Check sheet for the modelled part. Datum: model origin and axes. Units: mm. Face numbers are marked on the shaded views. Coordinates: 2 decimals unless noted, no trailing zeros. Loops run counter-clockwise (first coordinate to the right, second up) from the corner with the lowest first, then second, coordinate; pieces in that order, holes last. Notation, with made-up numbers: M 53,23 L 110,23 A22 ccw 110,58 Z; hole C 45.25,-2 d3. An arc over 180 degrees is marked long. Use CSV: the item, a comma, the result in double quotes. Start each with the question number.
(1) Section check A-A on x = -12.5. Record the cut outline in (y, z).
(2) Section check B-B on x = 14.5. Record the cut outline in (y, z), and give its area (3 significant figures).
(3) Scan lines: line 1 (X direction, y = 22, z = -14.75); line 2 (X direction, y = 18.75, z = -12.75); line 3 (X direction, y = 19.5, z = -10.5). Record each from-to range of solid material in increasing order.
(4) Go/stop test with flat-tipped pins: pin 1 Ø2 at (x, z) = (-14.5, -13) entering from -Y; pin 2 Ø3 at (x, z) = (-8.5, -17) entering from +Y; pin 3 Ø1 at (x, z) = (-9.5, -15) entering from -Y. Record where each tip stops, or that it passes through.
(5) Draft check along Y on the marked faces 1, 2 and 3. Enter one of: pulls with the +Y half, pulls with the -Y half, needs draft (parallel to the pull), parting line crosses it, or undercut.
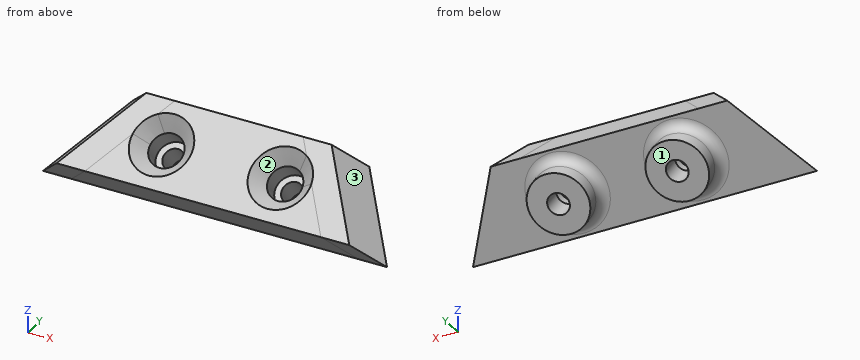
Autodesk Inventor part; units mm, degrees
ref_plane "作業平面2" through (-25, 27.5045, -21.6059) normal (0, -0.6427876, 0.7660444) x (1, 0, 0)
ref_plane "YZ Plane" through (0, 0, 0) normal (1, 0, 0) x (0, 1, 0)
ref_plane "XZ Plane" through (0, 0, 0) normal (0, 1, 0) x (-1, 0, 0)
sketch "スケッチ1" plane through (0, 0, 0) normal (0, 1, 0) x (-1, 0, 0)
  line L0 (28.2843, -28.2843) -> (0, 0)
  line L1 (0, 0) -> (-28.2843, -28.2843)
  line L2 (29.9813, -26.5872) -> (0, 3.3941)
  line L3 (0, 3.3941) -> (-29.9813, -26.5872)
  line L4 (28.2843, -28.2843) -> (29.9813, -26.5872)
  line L5 (-28.2843, -28.2843) -> (-29.9813, -26.5872)
  dimension "d0" = 40
  dimension "d1" = 2.4
extrude "押し出し1" add sketch "スケッチ1" along normal blind 50
sketch "スケッチ2" plane through (0, 0, 0) normal (1, 0, 0) x (0, 1, 0)
  line L0 (0, 3.3941) -> (31.9749, -34.7121)
  line L1 (0, 0) -> (0, -28.2843)
  line L2 (7.6604, 9.822) -> (39.6354, -28.2843)
  line L3 (0, 3.3941) -> (7.6604, 9.822)
  line L4 (39.6354, -28.2843) -> (31.9749, -34.7121)
  line L5 (0, -28.2843) -> (50, -28.2843)
  point P0 (26.5813, -28.2843)
  dimension "d4" = 40
  dimension "d5" = 10
extrude "押し出し2" cut sketch "スケッチ2" along normal mid plane 50 contours L3 L2 L5 L0 keep common part
ref_plane "作業平面1" through (0, 9.2239, 0.1802) normal (0, 0.7660444, 0.6427876) x (0.7938448, -0.3908923, 0.4658473)
sketch "スケッチ4" plane through (0, 9.2239, 0.1802) normal (0, 0.7660444, 0.6427876) x (0.7938448, -0.3908923, 0.4658473)
  line L0 (-37.1409, 7.3737) -> (2.5514, 37.7797)
  line L1 (-34.5895, 4.0431) -> (-39.6922, 10.7043)
  line L2 (0, 41.1103) -> (5.1027, 34.4491)
  point P0 (3.5216, -4.5971)
ref_plane "作業平面2" through (-25, 27.5045, -21.6059) normal (0, -0.6427876, 0.7660444) x (1, 0, 0)
sketch "スケッチ6" plane through (0, 9.2239, 0.1802) normal (0, 0.7660444, 0.6427876) x (0.7938448, -0.3908923, 0.4658473)
  line L0 (5.1027, -6.6611) -> (-34.5895, 4.0431)
  line L1 (5.1027, 34.4491) -> (5.1027, -6.6611)
  line L2 (5.1027, -6.6611) -> (-22.6818, 0.8318)
  line L3 (-22.6818, 0.8318) -> (5.1027, 22.116)
  line L4 (5.1027, 22.116) -> (5.1027, -6.6611)
  point P0 (3.5216, -4.5971)
  point P1 (5.1027, 22.116)
  dimension "d17" = 35
extrude "押し出し3" cut sketch "スケッチ6" along normal mid plane 50
sketch "スケッチ7" plane through (14.1059, 14.6842, -14.1059) normal (0, -0.6427876, 0.7660444) x (1, 0, 0)
  line L0 (3.3941, 0) -> (0, 0)
  line L1 (-3.0338, 10) -> (3.3941, 0)
  line L2 (-6.4279, 10) -> (-3.0338, 10)
  line L3 (-31.6059, 0) -> (-25.178, 10)
  line L4 (-28.2118, 0) -> (-31.6059, 0)
  line L5 (-21.7839, 10) -> (-28.2118, 0)
  line L6 (-25.178, 10) -> (-21.7839, 10)
  line L7 (-21.7839, 10) -> (-6.4279, 10)
  line L8 (-28.2118, 0) -> (0, 0)
  point P0 (-14.1059, -2.1817)
extrude "押し出し4" add sketch "スケッチ7" against normal blind 4
sketch "スケッチ10" plane through (-17.5, 14.6842, -14.1059) normal (0, -0.7660444, -0.6427876) x (1, 0, 0)
  line L0 (34.6701, -4) -> (42.5, -14.2213)
  line L1 (42.5, -9.7906) -> (42.5, -14.2213)
  line L2 (42.5, -9.7906) -> (35, 0)
  line L3 (0, 0) -> (-7.5, -9.7906)
  line L4 (-7.5, -14.2213) -> (-7.5, -9.7906)
  line L5 (-7.5, -14.2213) -> (0.3299, -4)
  line L6 (34.6701, -4) -> (0.3299, -4)
  line L7 (54.0058, -4) -> (-14.4099, -4)
  line L8 (-14.4099, -4) -> (-14.4099, -41.5974)
  line L9 (-14.4099, -41.5974) -> (54.0058, -41.5974)
  line L10 (54.0058, -41.5974) -> (54.0058, -4)
  point P0 (17.5, 20.2446)
  point P1 (-3.0642, -4)
  point P2 (38.0642, -4)
  point P3 (34.6701, -4)
extrude "押し出し6" cut sketch "スケッチ10" along normal through all both and the other way through all
sketch "スケッチ5" plane through (-25, 27.5045, -21.6059) normal (0, -0.6427876, 0.7660444) x (1, 0, 0)
  line L0 (0, 0) -> (50, 0)
  line L1 (17.9, 0) -> (32.1, 0)
  point P0 (25, -7.1817)
  point P1 (25, 0)
  dimension "d9" = 14.2
hole "穴1" at (-7.1, 27.5045, -21.6059) at (7.1, 27.5045, -21.6059) direction (0, -0.6427876, 0.7660444) diameter 4 end through all
sketch "スケッチ9" plane through (14.1059, 17.2554, -17.1701) normal (0, 0.6427876, -0.7660444) x (-1, 0, 0)
  circle A0 centre (21.2059, 5) radius 2 construction
  circle A1 centre (7.0059, 5) radius 2 construction
  circle A2 centre (7.0059, 5) radius 1.25
  circle A3 centre (7.0059, 5) radius 3.5
  circle A4 centre (21.2059, 5) radius 1.25
  circle A5 centre (21.2059, 5) radius 3.5
  point P0 (14.1059, -2.1817)
  dimension "d22" = 2.5
  dimension "d23" = 1.5
extrude "押し出し5" add sketch "スケッチ9" along normal blind 3
fillet "フィレット1" radius 1.2 2 edges at (-3.6, 21.0856, -13.9561) (10.6, 21.0856, -13.9561)
chamfer "面取り1" distance 1.6 angle 45 2 edges at (7.1, 16.9824, -12.1775) (-7.1, 16.9824, -12.1775)
properties part number "om_Drop_bumper"
Outcome:
1,outline,"M 14.68,-14.11 L 17.26,-17.17 L 24.92,-10.74 L 23.54,-9.11 L 20.64,-9.11 Z"
2,outline,"M 14.68,-14.11 L 17.26,-17.17 L 24.48,-11.11 L 18.26,-11.11 Z"
2,area,"28.2 mm²"
3,line 1,"x = -10.59 to -8.34, -5.86 to -3.61, 3.61 to 5.86, 8.34 to 10.59"
3,line 2,"x = -16.14 to -8.85, -5.35 to 5.35, 8.85 to 16.14"
3,line 3,"x = -13.89 to -10.21, -3.99 to 3.99, 10.21 to 13.89"
4,pin 1,"stops at y = 14.81"
4,pin 2,"stops at y = 23.91"
4,pin 3,"stops at y = 15.01"
5,face 1,"pulls with the +Y half"
5,face 2,"undercut"
5,face 3,"needs draft"
